Can you work these out from the model? Positions are in its coordinate system, mm. Face numbers are marked on the shaded views. A direction names the side the tool comes from. Coordinates: 2 decimals unless noted, no trailing zeros. Order: outer loops, then holes, each group sorted by start corner. A loop starts at its lowest first (then second) coordinate and runs counter-clockwise, first axis right, second up. Notation, with made-up numbers: (78, 28) - (82, 28) arc R13 ccw to (82, 52) - close; hole circle Ø11 at (18, 43.5). An arc over 180 degrees is marked (long way). Return JSON: item names as keys, results as strings. Group by question number.
1) Imagine slicing it at A-A (x = 0). Write out the boundary of the cut face in (y, z) (3 decimals).
2) Imagine slicing it at D-D (x = -13.5). Write out the boundary of the cut face in (y, z).
3) If we mould it in two halves opening along Z, with no side actions, what happens to the marked faces 5, 6, 7 and 8? For each: pulls with the +Z half, pulls with the -Z half, needs draft (parallel to the pull), parting line crosses it, or undercut.
4) For pin 1 Ø3 at (y, z) = (-21, 16.5) entering from +X; pin 2 Ø12.5 at (x, y) = (8, -11.5) entering from +Z; pin 3 Ø2 at (x, y) = (20, -5.5) entering from +Z; pin 4 Ø12 at (x, z) = (-34.5, 18.5) entering from -Y, each with a flat end and sliding along its axis, tell me the tip position at first contact or that it passes through.
5) If I drill on line 1 along Z through (x, y) = (0, -13.5) (3 decimals); line 2 along Z through (x, y) = (-13.5, -14); line 3 along Z through (x, y) = (0, -7.5) (3 decimals), over which ranges is the centre line in solid material (lowest first)?
6) Imagine slicing it at C-C (z = -13). Write out the boundary of the cut face in (x, y).
7) Which directions (+Z, -Z, +X, -X, +Y, -Y) give clear straight access to the entire face, cutting with the end or side of a thin tool? Please do the marked faces 1, 2, 3 and 4.
```python
from build123d import *

# Parameters (mm, degrees)
F0_R     = 31.75
F1_DEPTH = 25.4
F2_DEPTH = 12.7
F3_R     = 0.381


# Not quite as in the source:
# - a feature names something its author has since deleted; it is built from what else it names


with BuildPart() as f1:
    # F0 (on Front) → F1 (new body)
    with BuildSketch(Plane.XZ):
        with BuildLine():
            Line((15.3979316793, -36.83), (30.194233307, -36.83))
            ThreePointArc((30.194233307, -36.83), (42.108212504, -22.2494733583), (47.4402273678, -4.1911158763))
            Line((47.4402273678, -4.1911158763), (43.2608556704, -11.43))
            Line((43.2608556704, -11.43), (31.5290982004, -31.75))
            Line((31.5290982004, -31.75), (27.8629239911, -31.75))
            Line((27.8629239911, -31.75), (24.1967497817, -31.75))
            Line((24.1967497817, -31.75), (39.594681461, -5.08))
            Line((39.594681461, -5.08), (46.9928322749, 7.7339730917))
            ThreePointArc((46.9928322749, 7.7339730917), (40.3227154011, 25.3420450573), (27.349726503, 38.9888841237))
            Line((27.349726503, 38.9888841237), (30.6748353416, 33.2296266746))
            Line((30.6748353416, 33.2296266746), (34.095420147, 27.305))
            Line((34.095420147, 27.305), (43.2608556704, 11.43))
            Line((43.2608556704, 11.43), (41.4277685657, 8.255))
            Line((41.4277685657, 8.255), (39.594681461, 5.08))
            Line((39.594681461, 5.08), (26.7630717283, 27.305))
            Line((26.7630717283, 27.305), (25.1755740867, 30.0546265722))
            Line((25.1755740867, 30.0546265722), (16.7985989679, 44.5639730917))
            ThreePointArc((16.7985989679, 44.5639730917), (-1.7854971029, 47.5915184155), (-20.0905008648, 43.18))
            Line((-20.0905008648, 43.18), (-11.7317574699, 43.18))
            Line((-11.7317574699, 43.18), (11.7317574699, 43.18))
            Line((11.7317574699, 43.18), (13.5648445746, 40.005))
            Line((13.5648445746, 40.005), (15.3979316793, 36.83))
            Line((15.3979316793, 36.83), (-15.3979316793, 36.83))
            Line((-15.3979316793, 36.83), (-30.194233307, 36.83))
            ThreePointArc((-30.194233307, 36.83), (-42.108212504, 22.2494733583), (-47.4402273678, 4.1911158763))
            Line((-47.4402273678, 4.1911158763), (-44.833398728, 7.9780209084))
            Line((-44.833398728, 7.9780209084), (-31.5290982004, 27.305))
            Line((-31.5290982004, 27.305), (-27.2009059294, 27.305))
            Line((-27.2009059294, 27.305), (-22.8727136583, 27.305))
            Line((-22.8727136583, 27.305), (-38.6030217944, 4.4537921653))
            Line((-38.6030217944, 4.4537921653), (-46.9928322749, -7.7339730917))
            ThreePointArc((-46.9928322749, -7.7339730917), (-40.3227154011, -25.3420450573), (-27.349726503, -38.9888841237))
            Line((-27.349726503, -38.9888841237), (-31.5290982004, -31.75))
            Line((-31.5290982004, -31.75), (-43.2608556704, -11.43))
            Line((-43.2608556704, -11.43), (-41.4277685657, -8.255))
            Line((-41.4277685657, -8.255), (-39.594681461, -5.08))
            Line((-39.594681461, -5.08), (-24.1967497817, -31.75))
            Line((-24.1967497817, -31.75), (-16.7985989679, -44.5639730917))
            ThreePointArc((-16.7985989679, -44.5639730917), (1.7854971029, -47.5915184155), (20.0905008648, -43.18))
            Line((20.0905008648, -43.18), (11.7317574699, -43.18))
            Line((11.7317574699, -43.18), (-11.7317574699, -43.18))
            Line((-11.7317574699, -43.18), (-13.5648445746, -40.005))
            Line((-13.5648445746, -40.005), (-15.3979316793, -36.83))
            Line((-15.3979316793, -36.83), (15.3979316793, -36.83))
        make_face()
        Circle(F0_R, mode=Mode.SUBTRACT)
    extrude(amount=F1_DEPTH)

    # F0 (on Front) → F2 (join)
    with BuildSketch(Plane.XZ):
        Polygon((-41.7182102612, 6.2159065369), (-38.6030217944, 4.4537921653), (-22.8727136583, 27.305), (-27.2009059294, 27.305), align=None)
        Polygon((-44.833398728, 7.9780209084), (-41.7182102612, 6.2159065369), (-27.2009059294, 27.305), (-31.5290982004, 27.305), align=None)
        Polygon((-27.8629239911, -31.75), (-24.1967497817, -31.75), (-39.594681461, -5.08), (-41.4277685657, -8.255), align=None)
        Polygon((-31.5290982004, -31.75), (-27.8629239911, -31.75), (-41.4277685657, -8.255), (-43.2608556704, -11.43), align=None)
        Polygon((13.5648445746, -40.005), (15.3979316793, -36.83), (-15.3979316793, -36.83), (-13.5648445746, -40.005), align=None)
        Polygon((11.7317574699, -43.18), (13.5648445746, -40.005), (-13.5648445746, -40.005), (-11.7317574699, -43.18), align=None)
        Polygon((27.8629239911, -31.75), (41.4277685657, -8.255), (39.594681461, -5.08), (24.1967497817, -31.75), align=None)
        Polygon((31.5290982004, -31.75), (43.2608556704, -11.43), (41.4277685657, -8.255), (27.8629239911, -31.75), align=None)
        Polygon((43.2608556704, 11.43), (34.095420147, 27.305), (30.4292459376, 27.305), (41.4277685657, 8.255), align=None)
        Polygon((41.4277685657, 8.255), (30.4292459376, 27.305), (26.7630717283, 27.305), (39.594681461, 5.08), align=None)
        Polygon((13.5648445746, 40.005), (-13.5648445746, 40.005), (-15.3979316793, 36.83), (15.3979316793, 36.83), align=None)
        Polygon((11.7317574699, 43.18), (-11.7317574699, 43.18), (-13.5648445746, 40.005), (13.5648445746, 40.005), align=None)
    extrude(amount=F2_DEPTH)

    # F3
    f3_edges = [f1.edges().sort_by_distance(p)[0] for p in [
        (-47.440227, -12.7, 4.191116),
        (-27.349727, -12.7, -38.988884),
        (20.090501, -12.7, -43.18),
        (47.440227, -12.7, -4.191116),
        (27.349727, -12.7, 38.988884),
        (-20.090501, -12.7, 43.18),
    ]]
    fillet(f3_edges, radius=F3_R)


solid = f1.part
```
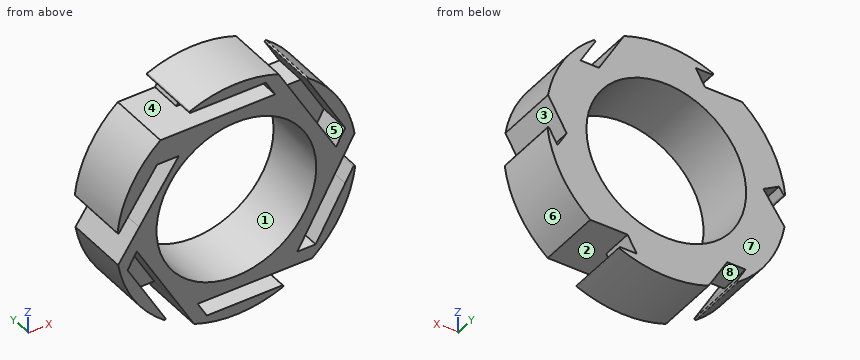
Calculated:
{
 "1": {"outline": "(-25.4, -47.625) - (0, -47.625) - (0, -31.75) - (-25.4, -31.75) - (-25.4, -36.83) - (-12.7, -36.83) - (-12.7, -43.18) - (-25.4, -43.18) - close; (-25.4, 31.75) - (0, 31.75) - (0, 47.625) - (-25.4, 47.625) - (-25.4, 43.18) - (-12.7, 43.18) - (-12.7, 36.83) - (-25.4, 36.83) - close"},
 "2": {"outline": "(-25.4, -45.67) - (0, -45.67) - (0, -28.74) - (-25.4, -28.74) - (-25.4, -36.83) - (-12.7, -36.83) - (-12.7, -40.12) - (-25.4, -40.12) - close; (-25.4, 28.74) - (0, 28.74) - (0, 40.12) - (-12.7, 40.12) - (-12.7, 36.83) - (-25.4, 36.83) - close; (-25.4, 43.18) - (0, 43.18) - (0, 45.67) - (-25.4, 45.67) - close"},
 "3": {"face 5": "undercut", "face 6": "pulls with the -Z half", "face 7": "needs draft", "face 8": "undercut"},
 "4": {"pin 1": "x = 45.2", "pin 2": "z = 47.59", "pin 3": "z = 40.75", "pin 4": "y = -25.4"},
 "5": {"line 1": "-47.625 to -43.18, -36.83 to -31.75, 31.75 to 36.83, 43.18 to 47.625", "line 2": "-45.67 to -40.12, -36.83 to -28.74, 28.74 to 36.83, 43.18 to 45.67", "line 3": "-47.625 to -31.75, 31.75 to 47.625"},
 "6": {"outline": "(-45.82, -25.4) - (-42.35, -25.4) - (-42.35, -12.7) - (-35.02, -12.7) - (-35.02, -25.4) - (-28.97, -25.4) - (-28.97, 0) - (-45.82, 0) - close; (28.97, -25.4) - (35.02, -25.4) - (35.02, -12.7) - (42.35, -12.7) - (42.35, -25.4) - (45.82, -25.4) - (45.82, 0) - (28.97, 0) - close"},
 "7": {"face 1": "+Y, -Y", "face 2": "+X, -Y", "face 3": "-Y", "face 4": "-X, -Y"}
}
